```python
from build123d import *

# Parameters (mm, degrees)
F0_R     = 3
F0_R_2   = 1.5
F0_R_3   = 5
F1_DEPTH = 4


with BuildPart() as f1:
    # F0 (on Right) → F1 (new body)
    with BuildSketch(Plane.YZ):
        with BuildLine():
            Line((-2.213923, 9.815771), (-50.172412, 4.496696))
            ThreePointArc((-50.172412, 4.496696), (-54.497093, -0.161719), (-49.848975, -4.497465))
            Line((-49.848975, -4.497465), (-19.228159, -1.781642))
            Line((-19.228159, -1.781642), (-10.071731, -4.497465))
            Line((-10.071731, -4.497465), (-4.982847, -21.569444))
            Line((-4.982847, -21.569444), (-4.982847, -70.413808))
            ThreePointArc((-4.982847, -70.413808), (-0.389649, -74.984794), (4.858025, -71.183044))
            Line((4.858025, -71.183044), (4.987747, -69.650171))
            Line((4.987747, -69.650171), (10.759941, -1.442462))
            ThreePointArc((10.759941, -1.442462), (10.680656, -0.04027), (10.214546, 1.284557))
            Line((10.214546, 1.284557), (8.115582, 5.324077))
            ThreePointArc((8.115582, 5.324077), (6.940309, 6.808469), (5.297374, 7.749453))
            Line((5.297374, 7.749453), (-0.044164, 9.577011))
            ThreePointArc((-0.044164, 9.577011), (-1.115855, 9.816243), (-2.213923, 9.815771))
        make_face()
        with Locations((0, -70)):
            Circle(F0_R, mode=Mode.SUBTRACT)
        with Locations((-50, 0)):
            Circle(F0_R_2, mode=Mode.SUBTRACT)
        Circle(F0_R_3, mode=Mode.SUBTRACT)
        with BuildLine():
            Line((4.987747, -69.650171), (4.858025, -71.183044))
            ThreePointArc((4.858025, -71.183044), (4.982191, -70.421626), (4.987747, -69.650171))
        make_face()
    extrude(amount=F1_DEPTH)


solid = f1.part
```
Here's how the part is built. I have some questions about the finished solid (model axes, mm). A direction names the side the tool comes from. Give positions to 0.01 mm unless a question says otherwise; leave off trailing zeros. Loops run counter-clockwise (first coordinate to the right, second up) from the corner with the lowest first, then second, coordinate; pieces in that order, holes last. Notation, with made-up numbers: M 21,39 L 73,39 A35 cw 73,71 Z; hole C 85.5,58.25 d7. An arc over 180 degrees is marked long. Put each result on its own line as item: value. Start each with the question number.
(1) I want a section at C-C on z = 0. Please give me the cut outline in (x, y), then the cut area to 3 significant figures.
(2) For faces 1 (the flat face through (1.97, -34.75, -3.16)), 2 (the flat face through (2, -4.983, -46)), 3 (the flat face through (1.972, 7.833, -36.024)), which set-ups out of +Z, -Z, +X, -X, +Y, -Y let a thin tool reach every point of the face, with its end or its side?
(3) I want a section at D-D on y = -33.5. Please give me the cut outline in (x, z), then the cut area to 3 significant figures.
(4) If we mould it in two halves opening along Y, with no side actions, what happens to faces 4 (the flat face through (1.972, -7.563, -12.914)), 5 (the flat face through (1.97, -14.71, -3.12)), 6 (the cylindrical face through (2, 0, -75))? For each: +Y half, -Y half, draft (parallel to the pull), parting line (faces both ways), or undercut.
(5) I want a section at B-B on y = 1.5. Please give me the cut outline in (x, z), then the cut area to 3 significant figures.
(6) I need wall thicknesses on line 1 along Z through (x, y) = (1.65, 0); line 2 along Z through (x, y) = (3.1, -50); line 3 along Y through (x, z) = (3.15, -70.5). Which ranges of each line are inside material? Lowest first, please. Write a range as [from, to].
(7) I want a section at A-A on x = 3.1. Please give me the cut outline in (y, z), then the cut area to 3 significant figures.
Answer block:
1. outline: M 0,-54.5 L 4,-54.5 L 4,-51.5 L 0,-51.5 Z; M 0,-48.5 L 4,-48.5 L 4,-5 L 0,-5 Z; M 0,5 L 4,5 L 4,10.67 L 0,10.67 Z
1. area: 209 mm^2
2. face 1: -Z, +X, -X
2. face 2: -Z, +X, -X, -Y
2. face 3: -Z, +X, -X, +Y
3. outline: M 0,-3.05 L 4,-3.05 L 4,6.35 L 0,6.35 Z
3. area: 37.6 mm^2
4. face 4: -Y half
4. face 5: undercut
4. face 6: parting line
5. outline: M 0,-74.77 L 4,-74.77 L 4,-72.6 L 0,-72.6 Z; M 0,-67.4 L 4,-67.4 L 4,-4.77 L 0,-4.77 Z; M 0,4.77 L 4,4.77 L 4,9.05 L 0,9.05 Z
5. area: 276 mm^2
6. line 1: [-75, -73], [-67, -5], [5, 9.56]
6. line 2: [-4.5, -1.5], [1.5, 4.52]
6. line 3: [-4.97, -2.96], [2.96, 4.97]
7. outline: M -50.17,4.5 A4.5 ccw -49.85,-4.5 L -19.23,-1.78 L -10.07,-4.5 L -4.98,-21.57 L -4.98,-70.41 A5 ccw 4.86,-71.18 A5 ccw 4.99,-69.65 L 10.76,-1.44 A5 ccw 10.21,1.28 L 8.12,5.32 A5 ccw 5.3,7.75 L -0.04,9.58 A5 ccw -2.21,9.82 Z; hole C -50,0 d3; hole C 0,0 d10; hole C 0,-70 d6
7. area: 1,490 mm^2
